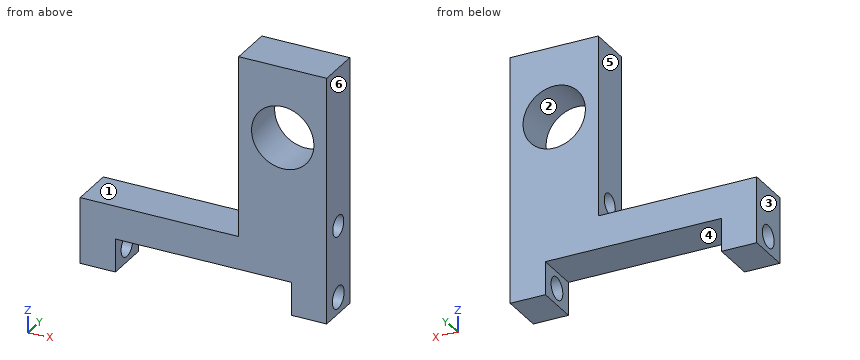
from build123d import *

# Parameters (mm, degrees)
SKETCH1_W             = 17.78
SKETCH1_H             = 17.78
BOSS_EXTRUDE1_DEPTH   = 3.175
SKETCH2_W             = 12.7
SKETCH2_H             = 4.7752
CUT_EXTRUDE1_DEPTH    = 4.175
F_8_CLEARANCE_HOLE1_D = 4.4958
F_0_CLEARANCE_HOLE1_D = 1.6129
F_1_72_TAPPED_HOLE1_D = 1.5113
SKETCH16_W            = 15.75311933
SKETCH16_H            = 13.574133519
CUT_EXTRUDE2_DEPTH    = 4.175


with BuildPart() as part:
    # Sketch1 → Boss-Extrude1 (new body)
    with BuildSketch(Plane(origin=(0, 0, 0), x_dir=(1, 0, 0), z_dir=(0, 1, 0))):
        Rectangle(SKETCH1_W, SKETCH1_H)
    extrude(amount=BOSS_EXTRUDE1_DEPTH)

    # Sketch2 → Cut-Extrude1 (cut, through all)
    with BuildSketch(Plane(origin=(0, 3.175, 0), x_dir=(1, 0, 0), z_dir=(0, 1, 0))):
        with Locations((0, 8.89)):
            Rectangle(SKETCH2_W, SKETCH2_H)
    extrude(amount=-CUT_EXTRUDE1_DEPTH, mode=Mode.SUBTRACT)

    # #8 Clearance Hole1 (through all)
    with Locations(Plane(origin=(0, 3.175, 0), x_dir=(1, 0, 0), z_dir=(0, 1, 0))):
        with Locations((5.715, -3.81)):
            Hole(F_8_CLEARANCE_HOLE1_D / 2)

    # #0 Clearance Hole1 (through all)
    with Locations(Plane(origin=(8.89, 0, 0), x_dir=(0, 0, -1), z_dir=(1, 0, 0))):
        with Locations((7.6962, 1.5875)):
            Hole(F_0_CLEARANCE_HOLE1_D / 2)

    # #1-72 Tapped Hole1 (through all)
    with Locations(Plane(origin=(8.89, 0, 0), x_dir=(0, 0, -1), z_dir=(1, 0, 0))):
        with Locations((2.54, 1.5875)):
            Hole(F_1_72_TAPPED_HOLE1_D / 2)

    # Sketch16 → Cut-Extrude2 (cut, through all)
    with BuildSketch(Plane(origin=(0, 3.175, 0), x_dir=(1, 0, 0), z_dir=(0, 1, 0))):
        with Locations((-5.336559665, -2.65956676)):
            Rectangle(SKETCH16_W, SKETCH16_H)
    extrude(amount=-CUT_EXTRUDE2_DEPTH, mode=Mode.SUBTRACT)


solid = part.part
Work out the finished part from the listing and answer in its coordinate system (mm). Face numbers are marked on the shaded views. A direction names the side the tool comes from. Give positions to 0.01 mm unless a question says otherwise; leave off trailing zeros. Order: outer loops, then holes, each group sorted by start corner. A loop starts at its lowest first (then second) coordinate and runs counter-clockwise, first axis right, second up. Notation, with made-up numbers: (64.25, -8.5) -> (102.25, -8.5) arc R27 cw to (102.25, 13.5) -> close; hole circle Ø5 at (28, 49.5). An arc over 180 degrees is marked (long way). Answer as a JSON object with one key per item and string values. Group by question number.
1. Consider line 1 along X through (y, z) = (2.5, -7); line 2 along Z through (x, y) = (-4.5, 1.85); line 3 along X through (y, z) = (0.2, -3.75). Determine where each line is inside the solid, lowest interval first. Write a range as [from, to].
2. Flat-ended cylindrical pins translate along their axes: pin 1 Ø1.5 at (x, z) = (-1.5, -3) entering from -Y; pin 2 Ø1 at (x, y) = (-2, 1.5) entering from -Z; pin 3 Ø1.5 at (y, z) = (1, 0.5) entering from -X; pin 4 Ø1.5 at (x, y) = (-1.5, 2.5) entering from +Z. Find the tip coordinate at first contact, or state that the pin passes through.
3. Section D-D on x = 7 is taken. Determine the outline of the cut face in (y, z) (1 decimal).
4. Section B-B on x = 4 is taken. Determine the outline of the cut face in (y, z) (1 decimal).
5. Section A-A on z = 3.81 is taken. Determine the outline of the cut face in (x, y) (3 decimals), plus the area to 3 significant figures.
6. A tool of negligible diameter and unlimited length cuts with its end or side. For the marked faces 5 and 6, from which of +Z, -Z, +X, -X, +Y, -Y can it reach the whole face along a straight path? Write none if from no direction.
7. The mould has two halves that part along X. Classify the marked faces 1, 2, 3 and 4: released by +X, released by -X, zero draft, split by the parting line, or undercut.
Result sheet:
{
 "1": {"line 1": "x = [-8.89, -6.35], [6.35, 8.89]", "line 2": "z = [-6.5, -4.13]", "line 3": "x = [2.54, 8.89]"},
 "2": {"pin 1": "passes through", "pin 2": "stops at z = -6.5", "pin 3": "stops at x = 2.54", "pin 4": "stops at z = -4.13"},
 "3": {"outline": "(0, -8.9) -> (3.2, -8.9) -> (3.2, 2) -> (0, 2) -> close; (0, 5.7) -> (3.2, 5.7) -> (3.2, 8.9) -> (0, 8.9) -> close; hole circle Ø1.6 at (1.6, -7.7); hole circle Ø1.5 at (1.6, -2.5)"},
 "4": {"outline": "(0, -6.5) -> (3.2, -6.5) -> (3.2, 2.4) -> (0, 2.4) -> close; (0, 5.3) -> (3.2, 5.3) -> (3.2, 8.9) -> (0, 8.9) -> close; hole circle Ø1.5 at (1.6, -2.5)"},
 "5": {"outline": "(2.54, 0) -> (3.467, 0) -> (3.467, 3.175) -> (2.54, 3.175) -> close; (7.963, 0) -> (8.89, 0) -> (8.89, 3.175) -> (7.963, 3.175) -> close", "area": "5.89 mm^2"},
 "6": {"face 5": "+Z, -X, +Y, -Y", "face 6": "+Z, -Z, +X, +Y, -Y"},
 "7": {"face 1": "zero draft", "face 2": "undercut", "face 3": "released by -X", "face 4": "undercut"}
}
